```python
from build123d import *

# Parameters (mm, degrees)
BOSS_EXTRUDE1_DEPTH = 25.4
SKETCH3_R           = 3.2004
CUT_EXTRUDE1_DEPTH  = 25.4


with BuildPart() as part:
    # Sketch2 → Boss-Extrude1 (new body)
    with BuildSketch(Plane.XY):
        Polygon((66.802, 0), (-66.802, 0), (-66.802, 6.985), (-64.262, 6.985), (-64.262, 5.08), (-38.608, 5.08), (-38.608, 6.985), (-36.068, 6.985), (-36.068, 5.08), (36.068, 5.08), (36.068, 6.985), (38.608, 6.985), (38.608, 5.08), (64.262, 5.08), (64.262, 6.985), (66.802, 6.985), align=None)
    extrude(amount=BOSS_EXTRUDE1_DEPTH)

    # Sketch3 → Cut-Extrude1 (cut)
    with BuildSketch(Plane(origin=(0, 5.08, 0), x_dir=(1, 0, 0), z_dir=(0, 1, 0))):
        with Locations(Location((-51.435, -12.7, 0), (0, 0, 270))):
            Circle(SKETCH3_R)
        with Locations(Location((51.435, -12.7, 0), (0, 0, 270))):
            Circle(SKETCH3_R)
    extrude(amount=-CUT_EXTRUDE1_DEPTH, mode=Mode.SUBTRACT)


solid = part.part
```
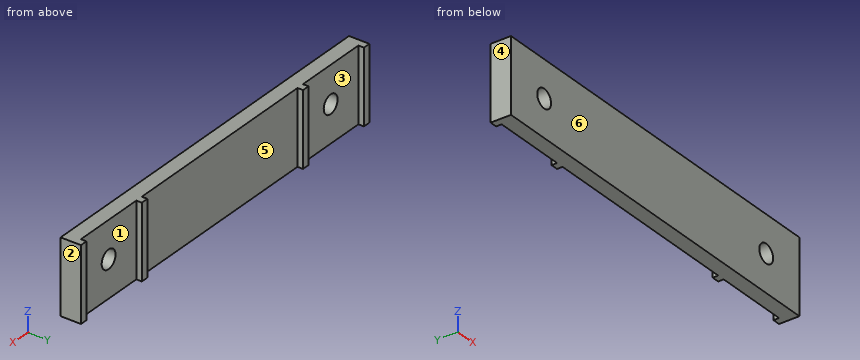
Geometry check sheet. Reference: the model listing, model coordinates, mm. Face numbers are marked on the shaded views. A direction names the side the tool comes from. Coordinates: 2 decimals unless noted, no trailing zeros. Loops run counter-clockwise (first coordinate to the right, second up) from the corner with the lowest first, then second, coordinate; pieces in that order, holes last. Notation, with made-up numbers: (-28.75, 76) - (10.25, 76) arc R21 cw to (10.25, 85) - close; hole circle Ø3 at (12.5, 56). An arc over 180 degrees is marked (long way). One line per item, written item: value. Start each with the question number.
(1) Cross-section at C-C on y = 4. Enter the section's corners in (x, z) (3 decimals), plus the area to 3 significant figures.
(2) Cross-section at D-D on x = 3.5. Enter the section's corners in (y, z), plus the area to 3 significant figures.
(3) Depth check by flat-ended pin: P1, Ø12, axis at x = 13.5, z = 16, coming from the +Y side. Enter the tip coordinate at first touch or a pass-through.
(4) Tool access check on the marked faces 1 and 2. Record the directions out of +Z, -Z, +X, -X, +Y, -Y that give a thin tool (end or side, any length) a straight path to the whole face; none if there is none.
(5) Cross-section at A-A on z = 12.7. Enter the section's corners in (x, y) (3 decimals).
(6) Cross-section at B-B on z = 18.25. Enter the section's corners in (x, y) (3 decimals).
(7) Mould release check, pull along X, two halves, no side actions. Record for the marked faces 3, 4, 5 and 6: released by +X, released by -X, zero draft, split by the parting line, or undercut.
(8) Material ranges on line 1 (X direction, y = 1.8, z = 12.7); line 2 (X direction, y = 6, z = 2.5); line 3 (X direction, y = 3.75, z = 10.5), recorded low to high. Write a range as [from, to].
Results below:
1. outline: (-66.802, 0) - (66.802, 0) - (66.802, 25.4) - (-66.802, 25.4) - close; hole circle Ø6.401 at (-51.435, 12.7); hole circle Ø6.401 at (51.435, 12.7)
1. area: 3,330 mm2
2. outline: (0, 0) - (5.08, 0) - (5.08, 25.4) - (0, 25.4) - close
2. area: 129 mm2
3. P1: stops at y = 5.08
4. face 1: +Z, -Z, +Y
4. face 2: +Z, -Z, +X, +Y, -Y
5. outline: (-66.802, 0) - (-54.635, 0) - (-54.635, 5.08) - (-64.262, 5.08) - (-64.262, 6.985) - (-66.802, 6.985) - close; (-48.235, 0) - (48.235, 0) - (48.235, 5.08) - (38.608, 5.08) - (38.608, 6.985) - (36.068, 6.985) - (36.068, 5.08) - (-36.068, 5.08) - (-36.068, 6.985) - (-38.608, 6.985) - (-38.608, 5.08) - (-48.235, 5.08) - close; (54.635, 0) - (66.802, 0) - (66.802, 6.985) - (64.262, 6.985) - (64.262, 5.08) - (54.635, 5.08) - close
6. outline: (-66.802, 0) - (66.802, 0) - (66.802, 6.985) - (64.262, 6.985) - (64.262, 5.08) - (38.608, 5.08) - (38.608, 6.985) - (36.068, 6.985) - (36.068, 5.08) - (-36.068, 5.08) - (-36.068, 6.985) - (-38.608, 6.985) - (-38.608, 5.08) - (-64.262, 5.08) - (-64.262, 6.985) - (-66.802, 6.985) - close
7. face 3: undercut
7. face 4: released by -X
7. face 5: undercut
7. face 6: zero draft
8. line 1: x = [-66.8, -54.64], [-48.23, 48.23], [54.64, 66.8]
8. line 2: x = [-66.8, -64.26], [-38.61, -36.07], [36.07, 38.61], [64.26, 66.8]
8. line 3: x = [-66.8, -53.76], [-49.11, 49.11], [53.76, 66.8]
